Design review of the part built by this model. Coordinates are the model's own, in mm. A direction names the side the tool comes from. Give positions to 0.01 mm unless a question says otherwise; leave off trailing zeros. Loops run counter-clockwise (first coordinate to the right, second up) from the corner with the lowest first, then second, coordinate; pieces in that order, holes last. Notation, with made-up numbers: (-22.5, -5) - (7.5, -5) arc R20 cw to (7.5, 16) - close; hole circle Ø7 at (41.5, -33). An arc over 180 degrees is marked (long way). Write each question's results on one line, items separated by ' | '.
```python
from build123d import *

# Parameters (mm, degrees)
SKETCH_1_R          = 8
SKETCH_1_R_2        = 1.25
EXTRUDE_1_DEPTH     = 12.5
SKETCH_3_R          = 1.75
CUT_EXTRUDE_1_DEPTH = 10
SKETCH_5_R          = 11.085638204
CUT_EXTRUDE_2_DEPTH = 1


with BuildPart() as part:
    # 草图1 → 凸台-拉伸1 (new body)
    with BuildSketch(Plane(origin=(0, 0, 0), x_dir=(1, 0, 0), z_dir=(0, 1, 0))):
        with Locations(Location((0, 0, 0), (0, 0, 270))):
            Circle(SKETCH_1_R)
        with Locations(Location((4.242640687, 4.242640687, 0), (0, 0, 270))):
            Circle(SKETCH_1_R_2, mode=Mode.SUBTRACT)
        with Locations(Location((4.242640687, -4.242640687, 0), (0, 0, 270))):
            Circle(SKETCH_1_R_2, mode=Mode.SUBTRACT)
        with Locations(Location((-4.242640687, -4.242640687, 0), (0, 0, 270))):
            Circle(SKETCH_1_R_2, mode=Mode.SUBTRACT)
        with Locations(Location((-4.242640687, 4.242640687, 0), (0, 0, 270))):
            Circle(SKETCH_1_R_2, mode=Mode.SUBTRACT)
        with BuildLine():
            Line((2.5, 1.658312395), (2.5, -1.658312395))
            ThreePointArc((2.5, -1.658312395), (-3, 0), (2.5, 1.658312395))
        make_face(mode=Mode.SUBTRACT)
    extrude(amount=EXTRUDE_1_DEPTH)

    # 草图3 → 切除-拉伸1 (cut)
    with BuildSketch(Plane.ZY.offset(-2.5)):
        with Locations((0, 6.5)):
            Circle(SKETCH_3_R)
    extrude(amount=-CUT_EXTRUDE_1_DEPTH, mode=Mode.SUBTRACT)

    # 草图5 → 切除-拉伸2 (cut)
    with BuildSketch(Plane.XZ):
        Circle(SKETCH_5_R)
    extrude(amount=-CUT_EXTRUDE_2_DEPTH, mode=Mode.SUBTRACT)


solid = part.part
```
Item 1: We need section C-C on y = 6.5. Give the boundary of the cut face in (x, z).
Output values:
outline: (2.5, -1.75) - (2.5, -1.66) arc R3 cw (long way) to (2.5, 1.66) - (2.5, 1.75) - (7.81, 1.75) arc R8 ccw (long way) to (7.81, -1.75) - close; hole circle Ø2.5 at (-4.24, -4.24); hole circle Ø2.5 at (-4.24, 4.24); hole circle Ø2.5 at (4.24, -4.24); hole circle Ø2.5 at (4.24, 4.24)
Item 2: We need section D-D on y = 9.5. Give the boundary of the cut face in (x, z).
Output values:
outline: circle Ø16 at (0, 0); hole circle Ø2.5 at (-4.24, -4.24); hole circle Ø2.5 at (-4.24, 4.24); hole (2.5, -1.66) - (2.5, 1.66) arc R3 ccw (long way) to start; hole circle Ø2.5 at (4.24, -4.24); hole circle Ø2.5 at (4.24, 4.24)
Item 3: Wall thickness on probe 1 along Z at (x, y) = (0, 7.75); probe 2 along Z at (x, y) = (4.5, 1.75); probe 3 along Z at (x, y) = (5, 7.75) (3 decimals): over which ranges is each line inside the solid? List them lowest first.
Output values:
probe 1: z = -8 to -3, 3 to 8 | probe 2: z = -6.61 to -5.47, -3.02 to 3.02, 5.47 to 6.61 | probe 3: z = -6.245 to -5.237, -3.248 to -1.225, 1.225 to 3.248, 5.237 to 6.245
Item 4: Tool access review of faces 4 (the face through (2.5, 3, 0)), 5 (the face through (5.21, 4.79, -0.38)), 6 (the face through (0.1, 12.5, 3.4)): name each direction out of +Z, -Z, +X, -X, +Y, -Y from which nothing blocks a thin tool from reaching the whole face with its end or side.
Output values:
face 4: +Y, -Y | face 5: +X | face 6: +Z, -Z, +X, -X, +Y
Item 5: Clearance check with flat-ended pins moving along their axes: P1, Ø4, axis at x = 4.24, z = -4.24, coming from the -Y side; P2, Ø4, axis at y = 5.5, z = -5, coming from the -X side; P3, Ø2, axis at y = 6.5, z = 0, coming from the +X side. State where each tip first meets the part, or that it passes through.
Output values:
P1: stops at y = 1 | P2: stops at x = -7.42 | P3: stops at x = -2.83
Item 6: We need section B-B on z = 1. Give the boundary of the cut face in (x, y).
Output values:
outline: (-7.94, 1) - (-2.83, 1) - (-2.83, 12.5) - (-7.94, 12.5) - close; (2.5, 1) - (7.94, 1) - (7.94, 5.06) - (2.5, 5.06) - close; (2.5, 7.94) - (7.94, 7.94) - (7.94, 12.5) - (2.5, 12.5) - close
Item 7: We need section A-A on x = 0. Give the boundary of the cut face in (y, z).
Output values:
outline: (1, -8) - (12.5, -8) - (12.5, -3) - (1, -3) - close; (1, 3) - (12.5, 3) - (12.5, 8) - (1, 8) - close
Item 8: Draft analysis for pull direction X (two halves, no side actions). For faces 1 (the face through (-7.81, 6.67, -1.73)), 2 (the face through (3, 1, 0)), 3 (the face through (3.134, 6.67, 4.819)), state which applies: +X half, -X half, draft (parallel to the pull), parting line (faces both ways), or undercut.
Output values:
face 1: parting line | face 2: draft | face 3: undercut
